Part model, mm, in its own coordinate system. Face numbers are marked on the shaded views. A direction names the side the tool comes from. Coordinates: 2 decimals unless noted, no trailing zeros. Order: outer loops, then holes, each group sorted by start corner. A loop starts at its lowest first (then second) coordinate and runs counter-clockwise, first axis right, second up. Notation, with made-up numbers: M 77,73 L 104,73 A38 ccw 104,112 Z; hole C 41.25,75 d6. An arc over 180 degrees is marked long. Write item = value, one per line. Start each with the question number.
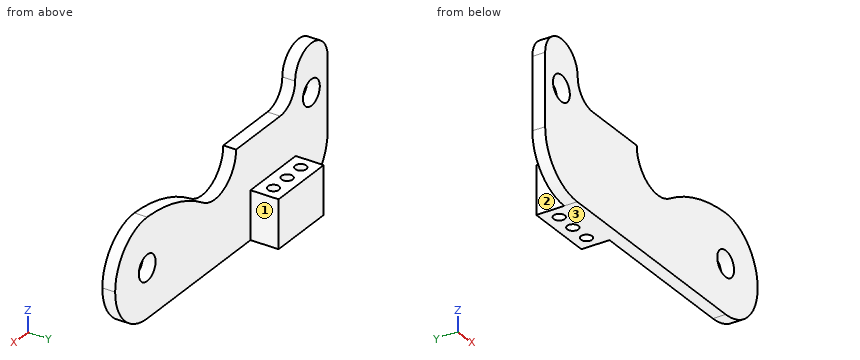
from build123d import *

# Parameters (mm, degrees)
BOSS_EXTRUDE1_DEPTH = 1.6
SKETCH4_R           = 1.6
CUT_EXTRUDE2_DEPTH  = 209.114814948
FILLET2_R           = 6.1
SKETCH2_W           = 8.6
SKETCH2_H           = 6
BOSS_EXTRUDE2_DEPTH = 3.5
CUT_EXTRUDE1_REACH  = 77.737
SKETCH3_R           = 0.7
FILLET1_R           = 20


# Some blends are built 0.0001 mm under size
with BuildPart() as part:
    # Sketch1 → Boss-Extrude1 (new body)
    with BuildSketch(Plane(origin=(0, 0, 0), x_dir=(1, 0, 0), z_dir=(0, 1, 0))):
        with BuildLine():
            Line((32.853134702, -176.602493772), (73.353134702, -176.602493772))
            Line((73.353134702, -176.602493772), (73.353134702, -188.802493772))
            Line((73.353134702, -188.802493772), (41.903134702, -188.802493772))
            ThreePointArc((41.903134702, -188.802493772), (39.887880375, -189.637239445), (39.053134702, -191.652493772))
            ThreePointArc((39.053134702, -191.652493772), (35.953134702, -194.752493772), (32.853134702, -191.652493772))
            Line((32.853134702, -191.652493772), (32.853134702, -176.602493772))
        make_face()
    extrude(amount=BOSS_EXTRUDE1_DEPTH)

    # Sketch4 → Cut-Extrude2 (cut, through all)
    with BuildSketch(Plane(origin=(0, 1.6, 0), x_dir=(1, 0, 0), z_dir=(0, 1, 0))):
        with Locations(Location((67.253134702, -182.702493772, 0), (0, 0, 270))):
            Circle(SKETCH4_R)
        with Locations(Location((35.953134702, -188.802493772, 0), (0, 0, 270))):
            Circle(SKETCH4_R)
        with BuildLine():
            Line((50.303134702, -188.802493772), (58.403134702, -188.802493772))
            ThreePointArc((58.403134702, -188.802493772), (54.353134702, -184.752493772), (50.303134702, -188.802493772))
        make_face()
    extrude(amount=-CUT_EXTRUDE2_DEPTH, mode=Mode.SUBTRACT)

    # Fillet2
    fillet2_edges = [part.edges().sort_by_distance(p)[0] for p in [
        (73.353134702, 0.8, 176.602493772),
        (73.353134702, 0.8, 188.802493772),
        (32.853134702, 0.8, 176.602493772),
    ]]
    fillet(fillet2_edges, radius=FILLET2_R - 0.0001)  # a hair under: the kernel refuses the full size

    # Sketch2 → Boss-Extrude2 (add)
    with BuildSketch(Plane(origin=(0, 1.6, 0), x_dir=(1, 0, 0), z_dir=(0, 1, 0))):
        with Locations((43.253134702, -179.602493772)):
            Rectangle(SKETCH2_W, SKETCH2_H)
    extrude(amount=BOSS_EXTRUDE2_DEPTH)

    # Sketch3 → Cut-Extrude1 (cut, up to next)
    with BuildSketch(Plane(origin=(0, 0, 176.602493772), x_dir=(-1, 0, 0), z_dir=(0, 0, -1)), mode=Mode.PRIVATE) as cut_extrude1_sk1:
        with Locations((-45.853134702, 3.35)):
            Circle(SKETCH3_R)
    cut_extrude1_tool1 = extrude(cut_extrude1_sk1.sketch, amount=-CUT_EXTRUDE1_REACH, mode=Mode.PRIVATE) & part.part
    # Sketch3 → Cut-Extrude1 (cut, up to next)
    with BuildSketch(Plane(origin=(0, 0, 176.602493772), x_dir=(-1, 0, 0), z_dir=(0, 0, -1)), mode=Mode.PRIVATE) as cut_extrude1_sk2:
        with Locations((-40.653134702, 3.35)):
            Circle(SKETCH3_R)
    cut_extrude1_tool2 = extrude(cut_extrude1_sk2.sketch, amount=-CUT_EXTRUDE1_REACH, mode=Mode.PRIVATE) & part.part
    # Sketch3 → Cut-Extrude1 (cut, up to next)
    with BuildSketch(Plane(origin=(0, 0, 176.602493772), x_dir=(-1, 0, 0), z_dir=(0, 0, -1)), mode=Mode.PRIVATE) as cut_extrude1_sk3:
        with Locations((-43.253134702, 3.35)):
            Circle(SKETCH3_R)
    cut_extrude1_tool3 = extrude(cut_extrude1_sk3.sketch, amount=-CUT_EXTRUDE1_REACH, mode=Mode.PRIVATE) & part.part
    add(cut_extrude1_tool1.solids().sort_by_distance((45.853135, 3.35, 176.602494))[0], mode=Mode.SUBTRACT)
    add(cut_extrude1_tool2.solids().sort_by_distance((40.653135, 3.35, 176.602494))[0], mode=Mode.SUBTRACT)
    add(cut_extrude1_tool3.solids().sort_by_distance((43.253135, 3.35, 176.602494))[0], mode=Mode.SUBTRACT)

    # Fillet1
    # the kernel refuses this fillet: 20 mm, written as the material it takes off along each edge
    with BuildSketch(Plane(origin=(58.403134702, 23.72525, 188.802493772), x_dir=(-0.4713226848050216, 0, -0.8819608419811995), z_dir=(0, -1, 0))) as fillet1_piece_1:
        with BuildLine():
            CenterArc((13.244167443, 17.63921684), FILLET1_R, 209.451639401, 32.428171428)
            Line((-4.171252893, 7.805441648), (-4.5195613, 7.608766144))
            ThreePointArc((-4.5195613, 7.608766144), (-2.438410783, 3.71419175), (-0.352784337, -0.188529074))
            Line((-0.352784337, -0.188529074), (0.188529074, -0.352784337))
            ThreePointArc((0.188529074, -0.352784337), (1.908856873, 0.07805859), (3.629184673, -0.352784337))
            Line((3.629184673, -0.352784337), (3.817713747, 0))
        make_face()
    extrude(amount=45.8505, mode=Mode.SUBTRACT)


solid = part.part
Item 1: Cut at A-A, the plane y = 3.35. Write the cut outline in (x, z), and give its area (3 significant figures).
Item 2: Flat gauge pins, fed straight in: pin 1 (1 mm diameter, centred on y = 3.5, z = 180.5, fed in from -X); pin 2 (1.8 mm diameter, centred on x = 45, y = 0.5, fed in from +Z); pin 3 (1 mm diameter, centred on y = 2, z = 184.5, fed in from -X); pin 4 (1.7 mm diameter, centred on x = 41, y = 4, fed in from +Z). Where does each tip first touch, or does it go through?
Item 3: Wall check: line 1 along Y through (x, z) = (52, 179.5); line 2 along X through (y, z) = (2.2, 178); line 3 along X through (y, z) = (1.15, 183.5). Give the ranges that are in metal, low to high. Write a range as [from, to].
Item 4: 3-axis set-ups, long thin cutter, end or side, ignore diameter. For the marked faces 1, 2 and 3: which of +Z, -Z, +X, -X, +Y, -Y reach the whole face in a straight line?
Item 5: Cut at D-D, the plane x = 52.5. Write the cut outline in (y, z).
Item 6: Cut at B-B, the plane z = 189.5. Write the cut outline in (x, y), and give its area (3 significant figures).
Item 7: Cut at C-C, the plane y = 1.15. Count the separate pieces of the cut face and the enclosed holes in it, and give its area (3 significant figures).
Filled sheet:
q1.outline = M 38.95,176.6 L 39.95,176.6 L 39.95,182.6 L 38.95,182.6 Z; M 41.35,176.6 L 42.55,176.6 L 42.55,182.6 L 41.35,182.6 Z; M 43.95,176.6 L 45.15,176.6 L 45.15,182.6 L 43.95,182.6 Z; M 46.55,176.6 L 47.55,176.6 L 47.55,182.6 L 46.55,182.6 Z
q1.area = 26.4 mm2
q2.pin_1 = 38.95
q2.pin_2 = 188.8
q2.pin_3 = 32.85
q2.pin_4 = 182.6
q3.line_1 = [0, 1.6]
q3.line_2 = [38.95, 47.55]
q3.line_3 = [32.85, 65.87], [68.64, 73.3]
q4.face_1 = +Z, -Z, +X, +Y
q4.face_2 = +Z, -Z, -X, +Y
q4.face_3 = -Z, +X, -X, +Y, -Y
q5.outline = M 0,176.6 L 1.6,176.6 L 1.6,185.2 L 0,185.2 Z
q6.outline = M 32.85,0 L 34.51,0 L 34.51,1.6 L 32.85,1.6 Z; M 37.39,0 L 40.04,0 L 40.04,1.6 L 37.39,1.6 Z
q6.area = 6.88 mm2
q7.separate_pieces = 1
q7.enclosed_holes = 2
q7.area = 455 mm2
